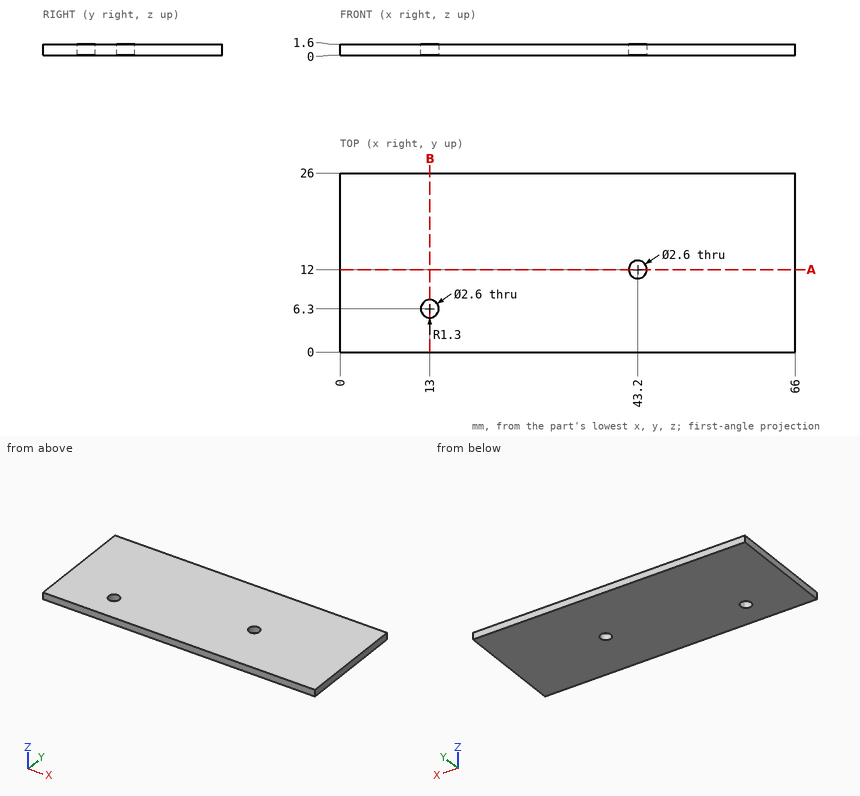
Geometry check sheet. Reference: drawing and pictorial views, mm from the part's lowest x, y, z. Round coordinates to 2 decimals unless told otherwise and drop trailing zeros. Write each loop counter-clockwise with the first axis right and the second up, starting at its lowest first coordinate (ties: lowest second). Pieces come first, ordered by that corner, then holes.
1. Scan lines: L1, parallel to Y at x = 13, z = 0.45; L2, parallel to Y at x = 43.2, z = 0.55; L3, parallel to X at y = 6.3, z = 0.8. Record each from-to range of solid material in increasing order.
2. Section check A-A on y = 12. Enter the section's corners in (x, z).
3. Gauge pin test, flat end, axial feed: P1, Ø4, axis at x = 38.5, y = 20.5, coming from the -Z side. Record the tip position at first contact, or that the pin passes through.
4. Section check B-B on x = 13. Enter the section's corners in (y, z), plus the area to 3 significant figures.
Answer:
1. L1: y = 0 to 5, 7.6 to 26
1. L2: y = 0 to 10.7, 13.3 to 26
1. L3: x = 0 to 11.7, 14.3 to 66
2. outline: (0, 0) - (41.9, 0) - (41.9, 1.6) - (0, 1.6) - close; (44.5, 0) - (66, 0) - (66, 1.6) - (44.5, 1.6) - close
3. P1: stops at z = 0
4. outline: (0, 0) - (5, 0) - (5, 1.6) - (0, 1.6) - close; (7.6, 0) - (26, 0) - (26, 1.6) - (7.6, 1.6) - close
4. area: 37.4 mm2
